Part model, mm, in its own coordinate system. A direction names the side the tool comes from. Give positions to 0.01 mm unless a question says otherwise; leave off trailing zeros. Write each loop counter-clockwise with the first axis right and the second up, starting at its lowest first coordinate (ties: lowest second). Pieces come first, ordered by that corner, then holes.
from build123d import *

# Parameters (mm, degrees)
SKETCH1_W           = 9.525
SKETCH1_H           = 14.351
BOSS_EXTRUDE1_DEPTH = 3.048
SKETCH2_W           = 4.7625
SKETCH2_H           = 8.001
BOSS_EXTRUDE2_DEPTH = 2.54
CHAMFER1_SIZE       = 1.27
CHAMFER2_SIZE       = 0.508
CHAMFER2_SIZE2      = 2.881011164


with BuildPart() as part:
    # Sketch1 → Boss-Extrude1 (new body)
    with BuildSketch(Plane.XY):
        with Locations((4.7625, -7.1755)):
            Rectangle(SKETCH1_W, SKETCH1_H)
    extrude(amount=BOSS_EXTRUDE1_DEPTH)

    # Sketch2 → Boss-Extrude2 (add)
    with BuildSketch(Plane.XY.offset(3.048)):
        with Locations((4.7625, -7.1755)):
            Rectangle(SKETCH2_W, SKETCH2_H)
    extrude(amount=BOSS_EXTRUDE2_DEPTH)

    # Chamfer1
    chamfer1_edges = [part.edges().sort_by_distance(p)[0] for p in [
        (4.7625, -3.175, 5.588),
    ]]
    chamfer(chamfer1_edges, length=CHAMFER1_SIZE)

    # Chamfer2
    chamfer2_edges = [part.edges().sort_by_distance(p)[0] for p in [
        (4.7625, 0, 3.048),
    ]]
    chamfer2_side = [part.faces().sort_by_distance(p)[0] for p in [
        (4.7625, 0, 1.524),
    ]]
    chamfer(chamfer2_edges, length=CHAMFER2_SIZE, length2=CHAMFER2_SIZE2, reference=chamfer2_side[0])


solid = part.part
1) Saw through at C-C (x = 1). Write the cut outline in (y, z), and give its area (3 significant figures).
Check result:
outline: (-14.35, 0) - (0, 0) - (0, 2.54) - (-2.88, 3.05) - (-14.35, 3.05) - close
area: 43.0 mm2
2) Saw through at A-A (y = -5.25). Write the cut outline in (x, z) (3 decimals), and give its area (3 significant figures).
Check result:
outline: (0, 0) - (9.525, 0) - (9.525, 3.048) - (7.144, 3.048) - (7.144, 5.588) - (2.381, 5.588) - (2.381, 3.048) - (0, 3.048) - close
area: 41.1 mm2
3) Drill centre lines: L1, parallel to X at y = -4.75, z = 4.35; L2, parallel to Z at x = 9, y = -4.5; L3, parallel to Y at x = 5, z = 4.15 (3 decimals). Where is each one in solid material? Low to high.
Check result:
L1: x = 2.38 to 7.14
L2: z = 0 to 3.05
L3: y = -11.176 to -3.175
4) 3-axis set-ups, long thin cutter, end or side, ignore diameter. For faces 1 (the flat face through (2.381, -7, 4)), 2 (the flat face through (5, -11.176, 4)), 3 (the flat face through (5, -14.351, 2)), 4 (the flat face through (5, -3.175, 4)), 5 (the flat face through (7.144, -7, 4)): which of +Z, -Z, +X, -X, +Y, -Y reach the whole face in a straight line?
Check result:
face 1: +Z, -X, +Y, -Y
face 2: +Z, +X, -X, -Y
face 3: +Z, -Z, +X, -X, -Y
face 4: +Z, +X, -X, +Y
face 5: +Z, +X, +Y, -Y
5) Flat gauge pins, fed straight in: P1, Ø2, axis at x = 5, z = 5, coming from the -Y side; P2, Ø0.8, axis at y = -7.5, z = 4, coming from the -X side; P3, Ø1, axis at x = 5.5, z = 4, coming from the +Y side (3 decimals). Where does each tip first touch, or does it go through?
Check result:
P1: stops at y = -11.18
P2: stops at x = 2.38
P3: stops at y = -3.175
6) Saw through at B-B (x = 5.75). Write the cut outline in (y, z) (3 decimals).
Check result:
outline: (-14.351, 0) - (0, 0) - (0, 2.54) - (-2.881, 3.048) - (-3.175, 3.048) - (-3.175, 4.318) - (-4.445, 5.588) - (-11.176, 5.588) - (-11.176, 3.048) - (-14.351, 3.048) - close
7) Saw through at D-D (z = 3.75). Write the cut outline in (x, y) (3 decimals).
Check result:
outline: (2.381, -11.176) - (7.144, -11.176) - (7.144, -3.175) - (2.381, -3.175) - close
